Autodesk Fusion 360 part; units mm, degrees
sketch "Sketch1" plane through (0, 0, 0) normal (0, 0, 1) x (1, 0, 0)
  line L0 (0, 0) -> (0, 38.1)
  line L1 (0, 38.1) -> (41.91, 38.1)
  line L2 (41.91, 38.1) -> (41.91, 0)
  line L3 (41.91, 0) -> (0, 0)
  dimension "d1" = 38.1
  dimension "d2" = 41.91
extrude "Extrude1" add sketch "Sketch1" along normal blind 2
sketch "Sketch3" plane through (0, 0, 2) normal (0, 0, 1) x (-1, 0, 0)
  line L0 (-41.91, 0) -> (-41.91, -38.1)
  line L1 (-41.91, -38.1) -> (0, -38.1)
  line L2 (0, -38.1) -> (0, 0)
  line L3 (0, 0) -> (-41.91, 0)
  circle A0 centre (-13.335, -9.525) radius 4.191
  line L4 (-13.335, -9.525) -> (-13.335, -38.1) construction
  line L5 (-13.335, -9.525) -> (-41.91, -9.525) construction
  dimension "d8" = 28.575
  dimension "d9" = 28.575
  dimension "d10" = 8.382
extrude "Extrude3" cut sketch "Sketch3" against normal blind 27.94 contours A0
sketch "Sketch4" plane through (0, 0, 2) normal (0, 0, 1) x (-1, 0, 0)
  circle A0 centre (-13.335, -9.525) radius 4.191
  line L0 (-41.91, 0) -> (-41.91, -38.1)
  line L1 (-41.91, -38.1) -> (0, -38.1)
  line L2 (0, -38.1) -> (0, 0)
  line L3 (0, 0) -> (-41.91, 0)
  line L4 (-12.7, -3.81) -> (-3.81, -3.81)
  line L5 (-12.7, -3.81) -> (-36.4901, -3.81)
  line L6 (-3.81, -34.29) -> (-3.81, -3.81)
  line L7 (-3.81, -34.29) -> (-36.4901, -34.29)
  line L8 (-36.4901, -34.29) -> (-36.4901, -3.81)
  dimension "d13" = 3.81
  dimension "d14" = 3.81
sketch "Sketch5" plane through (0, 0, 2) normal (0, 0, 1) x (-1, 0, 0)
sketch "Sketch6" plane through (0, 0, 2) normal (0, 0, 1) x (-1, 0, 0)
  line L0 (-13.3454, -9.4898) -> (-13.3454, -1.9898)
  line L1 (-13.3454, -9.4898) -> (-13.3454, -16.9898)
  line L2 (-13.3454, -16.9898) -> (-6.8454, -16.9898)
  line L3 (-13.3454, -16.9898) -> (-19.8454, -16.9898)
  line L4 (-6.8454, -16.9898) -> (-6.8454, -1.9898)
  line L5 (-6.8454, -1.9898) -> (-19.8454, -1.9898)
  line L6 (-19.8454, -16.9898) -> (-19.8454, -1.9898)
  line L7 (-6.8454, -18.9898) -> (-21.8454, -18.9898)
  line L8 (-21.8454, -1.9898) -> (-21.8454, -18.9898)
  line L9 (-19.8454, 0.0102) -> (-21.844, 0.0102)
  line L10 (-21.844, 0.0102) -> (-21.8454, -1.9898)
  line L11 (-19.8454, 0.0102) -> (-4.8454, 0.0102)
  line L12 (-6.8454, -18.9898) -> (-6.8454, -18.796)
  line L13 (-6.8454, -18.9898) -> (-4.8454, -18.9898)
  line L14 (-4.8454, -18.9898) -> (-4.8454, 0.0102)
  line L15 (-19.8454, -1.9898) -> (-20.32, -1.9898)
  line L16 (-20.32, -1.9898) -> (-21.8454, -1.9898)
  line L17 (-6.8454, -16.9898) -> (-6.8454, -18.9898)
  dimension "d15" = 7.5
  dimension "d16" = 7.5
  dimension "d17" = 6.5
  dimension "d18" = 6.5
  dimension "d19" = 15
  dimension "d20" = 13
  dimension "d21" = 2
  dimension "d22" = 2
  dimension "d23" = 2
  dimension "d24" = 2
sketch "Sketch8" plane through (0, 0, 2) normal (0, 0, 1) x (-1, 0, 0)
  line L0 (0, -34.29) -> (-41.91, -34.29)
  line L1 (0, -34.29) -> (0, -38.1)
  line L2 (0, -38.1) -> (-41.91, -38.1)
  line L3 (-41.91, -38.1) -> (-41.91, -34.29)
extrude "Extrude4" cut sketch "Sketch8" against normal blind 2.54
sketch "Sketch9" plane through (0, 0, 2) normal (0, 0, 1) x (-1, 0, 0)
  line L0 (0, 0) -> (0, 4)
  line L1 (0, 4) -> (-41.9328, 4)
  line L2 (-41.9328, 4) -> (-41.9328, 0)
  line L3 (-41.9328, 0) -> (0, 0)
  dimension "d27" = 4
extrude "Extrude5" add sketch "Sketch9" against normal blind 2.032
sketch "Sketch10" plane through (0, 0, 2) normal (0, 0, 1) x (-1, 0, 0)
  line L0 (-7.62, -30.48) -> (-33.02, -30.48)
  line L1 (-33.02, -30.48) -> (-33.02, -22.86)
  line L2 (-33.02, -22.86) -> (-7.62, -22.86)
  line L3 (-7.62, -22.86) -> (-7.62, -30.48)
extrude "Extrude6" cut sketch "Sketch10" against normal blind 2.54
extrude "Extrude7" add sketch "Sketch6" along normal blind 3 contours L2 L3 L6 L7 L8 L12 L15 L16 L17
equation "d15 = 15 mm / 2"
equation "d16 = 15 mm / 2"
equation "d17 = 13 mm / 2"
equation "d18 = 13 mm / 2"
For this review, take the finished solid that the model builds, in its own axes (mm). A direction names the side the tool comes from. Coordinates: 2 decimals unless noted, no trailing zeros. Loops run counter-clockwise (first coordinate to the right, second up) from the corner with the lowest first, then second, coordinate; pieces in that order, holes last. Notation, with made-up numbers: (3.5, -12.75) - (38.5, -12.75) arc R32 cw to (38.5, 17.25) - close; hole circle Ø3 at (-8, 78). An arc over 180 degrees is marked (long way). Use a Markdown table: item, result. Add a question column.
Item 1: Mouldability with a two-part tool opening along Y and no side actions: class faces 1 (the face through (7.62, 27, 1)), 2 (the face through (20, 22.86, 1)), 3 (the face through (21.845, 10, 3)), 4 (the face through (14, 18.99, 3)) as pulls with the +Y half, pulls with the -Y half, needs draft (parallel to the pull), parting line crosses it, or undercut.
Item 2: We need section C-C (x = 11). Give the number of separate pieces and of enclosed holes in the cut face, and give its area (3 significant figures).
Item 3: We need section D-D (y = 4.5). Give the boundary of the cut face in (x, z).
Item 4: Tool access review of faces 5 (the face through (20, 30.48, 1)), 6 (the face through (19.845, 10, 3)), 7 (the face through (21, 1.99, 3)), 8 (the face through (6.845, 18, 3)), 9 (the face through (20, 13, 5)): name each direction out of +Z, -Z, +X, -X, +Y, -Y from which nothing blocks a thin tool from reaching the whole face with its end or side.
Item 5: Insertion check: pin 1 Ø1 at (y, z) = (18, 3.5) entering from -X; pin 2 Ø17 at (x, y) = (12.5, 22.5) entering from -Z; pin 3 Ø1.5 at (x, y) = (37, 17.5) entering from +Z. Each pin has a flat end and moves straight along its axis. Give the tip position at first contact, or say it passes through.
Item 6: We need section B-B (y = 10). Give the boundary of the cut face in (x, z), and give its area (3 significant figures).
Item 7: For line 1 (X direction, y = 24, z = 1.85); line 2 (Z direction, x = 31.5, y = 2.5); line 3 (X direction, y = 18.5, z = 2.6), list the stretches that pass through material, from the lowest coordinate up.
Results list:
| question | item | result |
|---|---|---|
| 1 | face 1 | undercut |
| 1 | face 2 | undercut |
| 1 | face 3 | needs draft |
| 1 | face 4 | pulls with the +Y half |
| 2 | separate pieces | 3 |
| 2 | enclosed holes | 0 |
| 2 | area | 53.5 mm^2 |
| 3 | outline | (0, 0) - (41.91, 0) - (41.91, 2) - (21.85, 2) - (21.85, 5) - (19.85, 5) - (19.85, 2) - (0, 2) - close |
| 4 | face 5 | +Z, -Z |
| 4 | face 6 | +Z, -X, -Y |
| 4 | face 7 | +Z, +X, -X, -Y |
| 4 | face 8 | +Z, -X, +Y, -Y |
| 4 | face 9 | +Z, +X, -X, +Y, -Y |
| 5 | pin 1 | stops at x = 6.85 |
| 5 | pin 2 | stops at z = 0 |
| 5 | pin 3 | stops at z = 2 |
| 6 | outline | (0, 0) - (9.17, 0) - (9.17, 2) - (0, 2) - close; (17.5, 0) - (41.91, 0) - (41.91, 2) - (21.85, 2) - (21.85, 5) - (19.85, 5) - (19.85, 2) - (17.5, 2) - close |
| 6 | area | 73.2 mm^2 |
| 7 | line 1 | x = 0 to 7.62, 33.02 to 41.91 |
| 7 | line 2 | z = 0 to 2 |
| 7 | line 3 | x = 6.85 to 21.85 |
